Verification items for the finished model (mm, model axes). Face numbers are marked on the shaded views. Coordinates: 2 decimals unless noted, no trailing zeros. Order: outer loops, then holes, each group sorted by start corner. A loop starts at its lowest first (then second) coordinate and runs counter-clockwise, first axis right, second up. Notation, with made-up numbers: (52.25, 15.5) -> (92.25, 15.5) arc R26 ccw to (92.25, 45.5) -> close; hole circle Ø6 at (65.5, 41.25). An arc over 180 degrees is marked (long way). Write item = value, one per line. Start each with the question number.
1. Cross-section at B-B on z = 0. Record the cut outline in (x, y), plus the area to 3 significant figures.
2. Thickness scan on line 1 along Y through (x, z) = (-5.2, 0); line 2 along X through (y, z) = (1.25, 3); line 3 along X through (y, z) = (1.5, 1.5). Record the ranges inside material, lowest first. Write a range as from..to.
3. Cross-section at D-D on y = 3.5. Record the cut outline in (x, z), plus the area to 3 significant figures.
4. Go/stop test with flat-tipped pins: P1, Ø1.5, axis at y = 5, z = 4.5, coming from the -X side; P2, Ø3, axis at x = -5.5, z = 2, coming from the -Y side; P3, Ø4, axis at x = -5, y = 3.5, coming from the -Z side. Record where each tip stops, or that it passes through.
5. Cross-section at C-C on y = 1. Record the cut outline in (x, z), plus the area to 3 significant figures.
6. Cross-section at A-A on x = 0. Record the cut outline in (y, z).
7. Release check for a two-part mould opening along Y. For the marked faces 1, 2 and 3 record: +Y half, -Y half, draft (parallel to the pull), parting line (faces both ways), or undercut.
Autodesk Inventor part; units mm, degrees
ref_plane "YZ Plane" through (0, 0, 0) normal (1, 0, 0) x (0, 1, 0)
ref_plane "XZ Plane" through (0, 0, 0) normal (0, 1, 0) x (-1, 0, 0)
ref_plane "XY Plane" through (0, 0, 0) normal (0, 0, 1) x (1, 0, 0)
sketch "Sketch1" plane through (0, 0, 0) normal (0, 1, 0) x (-1, 0, 0)
  circle A0 centre (0, 0) radius 7
  circle A1 centre (0, 0) radius 4
  dimension "d0" = 14
  dimension "d1" = 8
extrude "Extrusion1" add sketch "Sketch1" along normal blind 7
chamfer "Chamfer1" distance 0.2 angle 45 4 edges at (7, 7, 0) (4, 7, 0) (7, 0, 0) (4, 0, 0)
sketch "Sketch2" plane through (0, 0, 0) normal (0, 1, 0) x (-1, 0, 0)
  point P0 (0, 0)
sketch "Sketch3" plane through (0, 0, 0) normal (1, 0, 0) x (0, 1, 0)
  circle A0 centre (3.5, 0) radius 2
  line L0 (7, -4.2) -> (7, 4.2)
  point P0 (0, 0)
  dimension "d7" = 4
  dimension "d8" = 3.5
extrude "Extrusion2" cut sketch "Sketch3" against normal blind 7
properties part number "8mmShaftCollar"
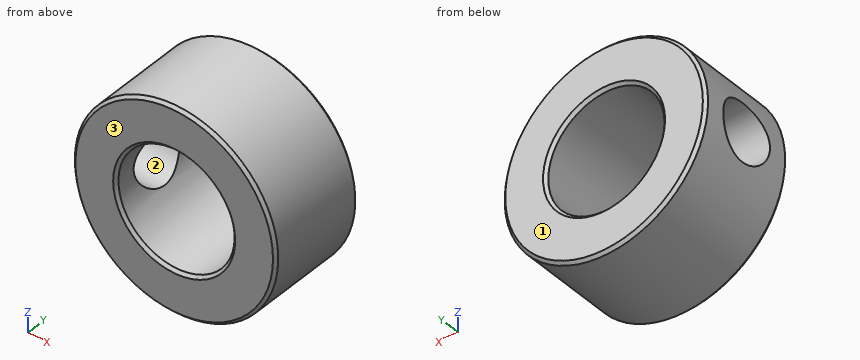
Worked out:
q1.outline = (-7, 0.2) -> (-6.8, 0) -> (-4.2, 0) -> (-4, 0.2) -> (-4, 1.5) -> (-7, 1.5) -> close; (-7, 5.5) -> (-4, 5.5) -> (-4, 6.8) -> (-4.2, 7) -> (-6.8, 7) -> (-7, 6.8) -> close; (4, 0.2) -> (4.2, 0) -> (6.8, 0) -> (7, 0.2) -> (7, 6.8) -> (6.8, 7) -> (4.2, 7) -> (4, 6.8) -> close
q1.area = 29.8 mm²
q2.line_1 = 0..1.5, 5.5..7
q2.line_2 = -6.32..-2.65, 2.65..6.32
q2.line_3 = -6.84..-3.71, 3.71..6.84
q3.outline = (-6.71, -2) arc R7 ccw (long way) to (-6.71, 2) -> (-3.46, 2) arc R4 cw (long way) to (-3.46, -2) -> close
q3.area = 91.4 mm²
q4.P1 = -5.91
q4.P2 = 0
q4.P3 = -6.32
q5.outline = circle Ø14 at (0, 0); hole circle Ø8 at (0, 0)
q5.area = 104 mm²
q6.outline = (0, -6.8) -> (0.2, -7) -> (6.8, -7) -> (7, -6.8) -> (7, -4.2) -> (6.8, -4) -> (0.2, -4) -> (0, -4.2) -> close; (0, 4.2) -> (0.2, 4) -> (6.8, 4) -> (7, 4.2) -> (7, 6.8) -> (6.8, 7) -> (0.2, 7) -> (0, 6.8) -> close
q7.face_1 = +Y half
q7.face_2 = undercut
q7.face_3 = -Y half
